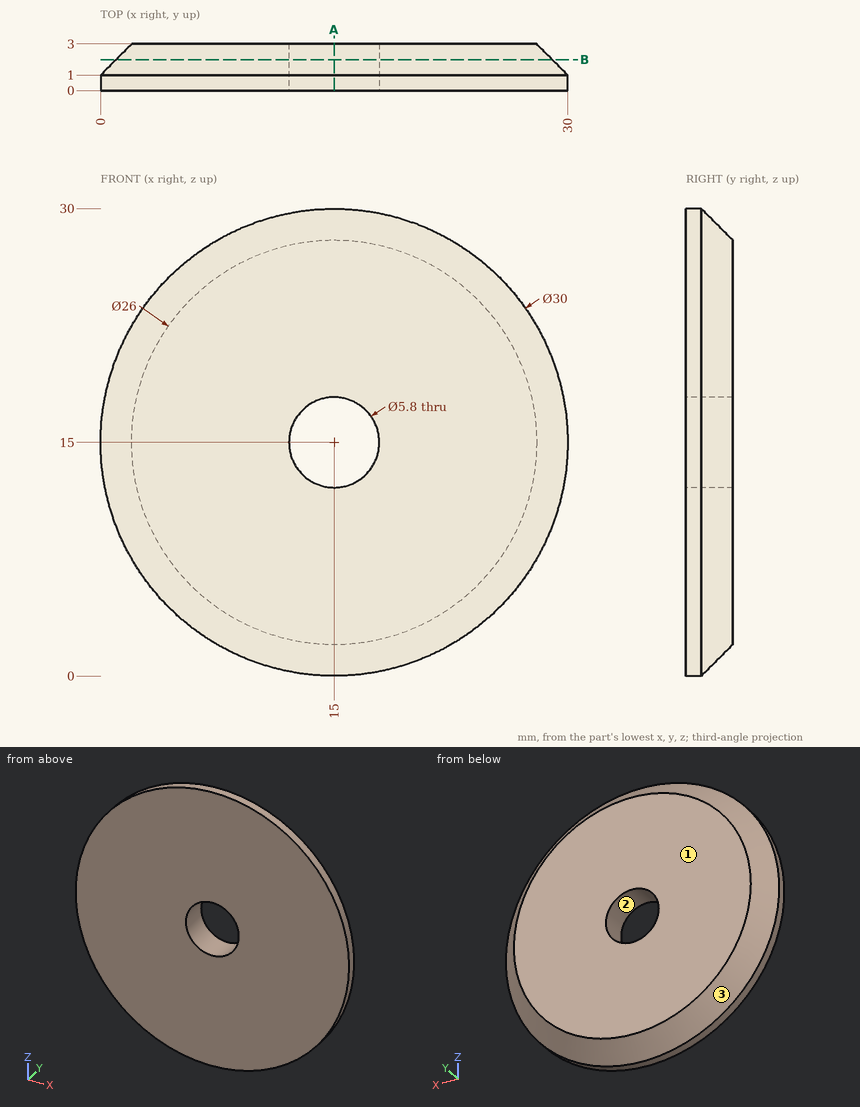
Print and shaded views of the part. All mm, measured from the part's lowest x, y and z. Coordinates: 2 decimals unless noted, no trailing zeros. Order: outer loops, then holes, each group sorted by start corner. A loop starts at its lowest first (then second) coordinate and runs counter-clockwise, first axis right, second up. Notation, with made-up numbers: M 38.25,-30 L 61.25,-30 A26 cw 61.25,-11 Z; hole C 67,-23 d9. An arc over 180 degrees is marked long. Write each question's results on one line, items separated by ' | '. Start each with the question number.
Q1. Pull direction Z, two halves, no side cores. Call the marked faces 1, 2 and 3: +Z half, -Z half, draft (parallel to the pull), parting line (faces both ways), or undercut.
Q2. Cut at B-B (y = 2). List the corners of the cut face in (x, z).
Q3. Flat gauge pins, fed straight in: P1, Ø1, axis at x = 9.5, y = 0.5, coming from the -Z side; P2, Ø1, axis at y = 2, z = 10.5, coming from the -X side. Where does each tip first touch, or does it go through?
Q4. Drill centre lines: probe 1 along Z at (x, y) = (15, 0.7); probe 2 along Z at (x, y) = (13.5, 2.65). Where is each one in solid material? Low to high. Write a range as from..to.
Q5. Cut at A-A (x = 15). List the corners of the cut face in (y, z).
Found:
1) face 1: draft | face 2: undercut | face 3: parting line
2) outline: C 15,15 d28; hole C 15,15 d5.8
3) P1: z = 0.86 | P2: x = 1.19
4) probe 1: 0..12.1, 17.9..30 | probe 2: 1.73..12.52, 17.48..28.27
5) outline: M 0,0 L 1,0 L 3,2 L 3,12.1 L 0,12.1 Z; M 0,17.9 L 3,17.9 L 3,28 L 1,30 L 0,30 Z
